CAD build for the part. Positions are in the model's coordinates, mm. A direction names the side the tool comes from. Round coordinates to 2 decimals unless told otherwise and drop trailing zeros. Write each loop counter-clockwise with the first axis right and the second up, starting at its lowest first coordinate (ties: lowest second). Pieces come first, ordered by that corner, then holes. Notation, with made-up numbers: M 55.5,10.5 L 75.5,10.5 A21 cw 75.5,46.5 Z; hole C 53.5,-30 d10. An arc over 180 degrees is marked long. Write each question's results on one line, items separated by ' | '. Start each with the question number.
```python
from build123d import *

# Parameters (mm, degrees)
SKETCH2_W           = 38
SKETCH2_H           = 38
SKETCH3_W           = 30
SKETCH3_H           = 30
SKETCH4_R           = 4
CUT_EXTRUDE1_DEPTH  = 1001.902093114
SWEEP2_PROFILE_R    = 2.5
CUT_EXTRUDE2_DEPTH  = 1003.203029253
BOSS_EXTRUDE1_DEPTH = 38
SKETCH22_W          = 30
SKETCH22_H          = 30
CUT_EXTRUDE3_DEPTH  = 1074.472400545
CUT_EXTRUDE4_DEPTH  = 1003.203029253
CUT_EXTRUDE5_DEPTH  = 1003.203029253
BOSS_EXTRUDE2_REACH = 1004.203


with BuildPart() as part:
    # Sweep1: sweep along a path in Sketch1
    with BuildLine(Plane(origin=(0, 0, 0), x_dir=(1, 0, 0), z_dir=(0, 1, 0))) as sweep1_path:
        Line((0, 0), (-1000, 0))
    # Sketch2 → Sweep1 (sweep)
    with BuildSketch(Plane(origin=(0, 0, 0), x_dir=(0, 0, -1), z_dir=(1, 0, 0))):
        Rectangle(SKETCH2_W, SKETCH2_H)
    sweep(path=sweep1_path.line)

    # Cut-Sweep1: sweep along a path in Sketch1_2
    with BuildLine(Plane(origin=(0, 0, 0), x_dir=(1, 0, 0), z_dir=(0, 1, 0))) as cut_sweep1_path:
        Line((0, 0), (-1000, 0))
    # Sketch3 → Cut-Sweep1 (sweep, cut)
    with BuildSketch(Plane(origin=(0, 0, 0), x_dir=(0, 0, -1), z_dir=(1, 0, 0))):
        Rectangle(SKETCH3_W, SKETCH3_H)
    sweep(path=cut_sweep1_path.line, mode=Mode.SUBTRACT)

    # Sketch4 → Cut-Extrude1 (cut, through all)
    with BuildSketch(Plane(origin=(0, 19, 0), x_dir=(1, 0, 0), z_dir=(0, 1, 0))):
        with Locations(Location((-212.63683242, 0, 0), (0, 0, 270))):
            Circle(SKETCH4_R)
    extrude(amount=-CUT_EXTRUDE1_DEPTH, mode=Mode.SUBTRACT)

    # Sweep2: sweep along a path in Sketch5
    with BuildLine(Plane.ZY.offset(985)) as sweep2_path:
        Line((-19, 0), (-26.570946825, 0))
        ThreePointArc((-26.570946825, 0), (-29.503401087, 0.950220747), (-31.321263798, 3.4397152))
        ThreePointArc((-31.321263798, 3.4397152), (-51.969366005, 0.135523131), (-31.321263798, -3.168668939))
    # Sweep2 profile (on start of the path) → Sweep2 (sweep)
    with BuildSketch(Plane(origin=(-985, 0, -19), x_dir=(0, -1, 0), z_dir=(0, 0, -1))):
        Circle(SWEEP2_PROFILE_R)
    sweep(path=sweep2_path.line)

    # Sketch16 → Cut-Extrude2 (cut, through all)
    with BuildSketch(Plane(origin=(0, 19, 0), x_dir=(1, 0, 0), z_dir=(0, 1, 0))):
        Polygon((0, -19), (0, 19), (-71.907398101, -19), align=None)
    extrude(amount=-CUT_EXTRUDE2_DEPTH, mode=Mode.SUBTRACT)

    # Sketch17 → Boss-Extrude1 (add)
    with BuildSketch(Plane(origin=(0, 19, 0), x_dir=(1, 0, 0), z_dir=(0, 1, 0))):
        Polygon((-71.907398101, -19), (0, -19), (71.921211139, 19), (0, 19), align=None)
    extrude(amount=-BOSS_EXTRUDE1_DEPTH)

    # Sketch22 → Cut-Extrude3 (cut, through all)
    with BuildSketch(Plane.ZY.offset(1000)):
        Rectangle(SKETCH22_W, SKETCH22_H)
    extrude(amount=-CUT_EXTRUDE3_DEPTH, mode=Mode.SUBTRACT)

    # Sketch23 → Cut-Extrude4 (cut, through all)
    with BuildSketch(Plane(origin=(0, 19, 0), x_dir=(1, 0, 0), z_dir=(0, 1, 0))):
        Polygon((14.258492684, 0), (-32.20683242, -19), (0, -19), (71.921211139, 19), (60.723817789, 19), align=None)
    extrude(amount=-CUT_EXTRUDE4_DEPTH, mode=Mode.SUBTRACT)

    # Sketch24 → Cut-Extrude5 (cut, through all)
    with BuildSketch(Plane(origin=(0, 19, 0), x_dir=(1, 0, 0), z_dir=(0, 1, 0))):
        Polygon((-78.672157524, -19), (14.258492684, 19), (60.723817789, 19), (-32.20683242, -19), align=None)
    extrude(amount=-CUT_EXTRUDE5_DEPTH, mode=Mode.SUBTRACT)

    # Sketch25 → Boss-Extrude2 (add, up to next)
    with BuildSketch(Plane(origin=(0, 19, 0), x_dir=(1, 0, 0), z_dir=(0, 1, 0)), mode=Mode.PRIVATE) as boss_extrude2_sk1:
        Polygon((3.690100071, 19), (-89.240550137, -19), (-78.672157524, -19), (14.258492684, 19), align=None)
    boss_extrude2_tool1 = extrude(boss_extrude2_sk1.sketch, amount=-BOSS_EXTRUDE2_REACH, mode=Mode.PRIVATE) - part.part
    add(boss_extrude2_tool1.solids().sort_by_distance((-37.491029, 19, 0))[0])


solid = part.part
```
1) 3-axis set-ups, long thin cutter, end or side, ignore diameter. For faces 1 (the face through (-510, 15, 0)), 2 (the face through (-32.857, 0.266, 0.266)): which of +Z, -Z, +X, -X, +Y, -Y reach the whole face in a straight line?
2) Wall check: line 1 along Z through (x, y) = (-615, -11); line 2 along X through (y, z) = (-16.5, 2.5). Give the ranges that are in metal, low to high. Write a range as from..to.
3) Drop flat-ended pins along their axis: pin 1 Ø5 at (y, z) = (1.5, -9.5) entering from -X; pin 2 Ø6 at (y, z) = (-13, -46.5) entering from -X; pin 3 Ø1.5 at (x, y) = (-192.5, -10.5) entering from -Z; pin 4 Ø13 at (x, z) = (-212.64, 0) entering from -Y. Give the stop position or say it passes through.
4) Pull direction Z, two halves, no side cores. Call faces 3 (the face through (-546, 0, 15)), 4 (the face through (-546, 0, 19)), 5 (the face through (-500, -19, 0)): pulls with the +Z half, pulls with the -Z half, needs draft (parallel to the pull), parting line crosses it, or undercut.
5) Saw through at A-A, the plane x = -551. Write the cut outline in (y, z).
Filled sheet:
1) face 1: -X | face 2: +Z, +X, +Y, -Y
2) line 1: z = -19..-15, 15..19 | line 2: x = -1000..-215.76, -209.51..-38.32
3) pin 1: stops at x = -25.66 | pin 2: stops at x = -987.45 | pin 3: stops at z = -19 | pin 4: stops at y = -19
4) face 3: undercut | face 4: pulls with the +Z half | face 5: needs draft
5) outline: M -19,-19 L 19,-19 L 19,19 L -19,19 Z; hole M -15,-15 L 15,-15 L 15,15 L -15,15 Z
